Build history of the part. All positions in model axes, mm. Face numbers are marked on the shaded views. A direction names the side the tool comes from. Give positions to 0.01 mm unless a question says otherwise; leave off trailing zeros. Order: outer loops, then holes, each group sorted by start corner. A loop starts at its lowest first (then second) coordinate and runs counter-clockwise, first axis right, second up. Notation, with made-up numbers: (69.5, -21.5) -> (88.5, -21.5) arc R22 ccw to (88.5, 14.5) -> close; hole circle Ø8 at (82, -16.5). An arc over 180 degrees is marked (long way). Use a Markdown table: item, result. Add a question column.
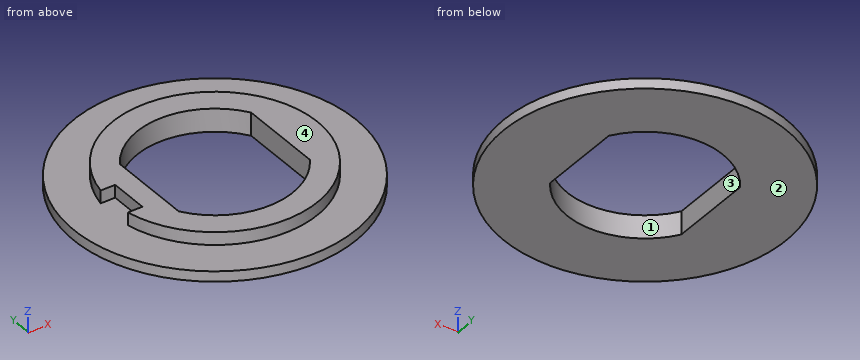
```python
from build123d import *

# Parameters (mm, degrees)
F0_R     = 17.4625
F1_DEPTH = 1.27
F3_DEPTH = 1.5748
F5_DEPTH = 2.8458


with BuildPart() as f1:
    # F0 (on Top) → F1 (new body)
    with BuildSketch(Plane.XY):
        Circle(F0_R)
    extrude(amount=F1_DEPTH)

    # F2 (on face) → F3 (join)
    with BuildSketch(Plane.XY.offset(1.27)):
        with BuildLine():
            Line((-10.668, -2.413), (-12.468658, -2.413))
            ThreePointArc((-12.468658, -2.413), (12.7, 0), (-12.468658, 2.413))
            Line((-12.468658, 2.413), (-10.668, 2.413))
            Line((-10.668, 2.413), (-10.668, -2.413))
        make_face()
    extrude(amount=F3_DEPTH)

    # F4 (on face) → F5 (cut, through all)
    with BuildSketch(Plane.XY.offset(2.8448)):
        with BuildLine():
            Line((-8.128, 5.205451), (-8.128, -5.205451))
            ThreePointArc((-8.128, -5.205451), (0, -9.652), (8.128, -5.205451))
            Line((8.128, -5.205451), (8.128, 5.205451))
            ThreePointArc((8.128, 5.205451), (0, 9.652), (-8.128, 5.205451))
        make_face()
    extrude(amount=-F5_DEPTH, mode=Mode.SUBTRACT)


solid = f1.part
```
(1) Band-saw the part on C-C on y = 0. Give the cut face in (x, z).
(2) Band-saw the part on A-A on z = 2.35. Give the cut face in (x, y), plus the area to 3 significant figures.
(3) Mould opens along Y. For the marked faces 3 and 4 say: released by +Y, released by -Y, zero draft, split by the parting line, or undercut.
(4) Pin check, flat tips, straight feed: pin 1 Ø0.8 at (x, z) = (-11.5, 2) entering from -Y; pin 2 Ø0.9 at (y, z) = (-1.5, 1) entering from -X; pin 3 Ø1.3 at (x, z) = (-11.5, 2) entering from +Y. Stop position of each tip, or through.
(5) Band-saw the part on D-D on z = 0.45. Give the cut face in (x, y) (1 decimal), plus the area to 3 significant figures.
(6) Band-saw the part on B-B on x = 0. Give the cut face in (y, z), plus the area to 3 significant figures.
(7) Wall check: probe 1 along Y at (x, z) = (0, 2.1); probe 2 along Y at (x, z) = (-3, 2.25); probe 3 along X at (y, z) = (-8, 1.6). Give the ranges that are in metal, low to high.
(8) Tool access for the marked faces 1 and 2: list every direction of +Z, -Z, +X, -X, +Y, -Y with a clear straight run to the whole face (end or side of a thin tool).
Response:
| question | item | result |
|---|---|---|
| 1 | outline | (-17.46, 0) -> (-8.13, 0) -> (-8.13, 2.84) -> (-10.67, 2.84) -> (-10.67, 1.27) -> (-17.46, 1.27) -> close; (8.13, 0) -> (17.46, 0) -> (17.46, 1.27) -> (12.7, 1.27) -> (12.7, 2.84) -> (8.13, 2.84) -> close |
| 2 | outline | (-12.47, -2.41) arc R12.7 ccw (long way) to (-12.47, 2.41) -> (-10.67, 2.41) -> (-10.67, -2.41) -> close; hole (-8.13, -5.21) arc R9.65 ccw to (8.13, -5.21) -> (8.13, 5.21) arc R9.65 ccw to (-8.13, 5.21) -> close |
| 2 | area | 226 mm² |
| 3 | face 3 | undercut |
| 3 | face 4 | zero draft |
| 4 | pin 1 | stops at y = -6.17 |
| 4 | pin 2 | stops at x = -17.43 |
| 4 | pin 3 | stops at y = 6.6 |
| 5 | outline | circle Ø34.9 at (0, 0); hole (-8.1, -5.2) arc R9.7 ccw to (8.1, -5.2) -> (8.1, 5.2) arc R9.7 ccw to (-8.1, 5.2) -> close |
| 5 | area | 687 mm² |
| 6 | outline | (-17.46, 0) -> (-9.65, 0) -> (-9.65, 2.84) -> (-12.7, 2.84) -> (-12.7, 1.27) -> (-17.46, 1.27) -> close; (9.65, 0) -> (17.46, 0) -> (17.46, 1.27) -> (12.7, 1.27) -> (12.7, 2.84) -> (9.65, 2.84) -> close |
| 6 | area | 29.4 mm² |
| 7 | probe 1 | y = -12.7 to -9.65, 9.65 to 12.7 |
| 7 | probe 2 | y = -12.34 to -9.17, 9.17 to 12.34 |
| 7 | probe 3 | x = -9.86 to -5.4, 5.4 to 9.86 |
| 8 | face 1 | +Z, -Z |
| 8 | face 2 | -Z, +X, -X, +Y, -Y |
